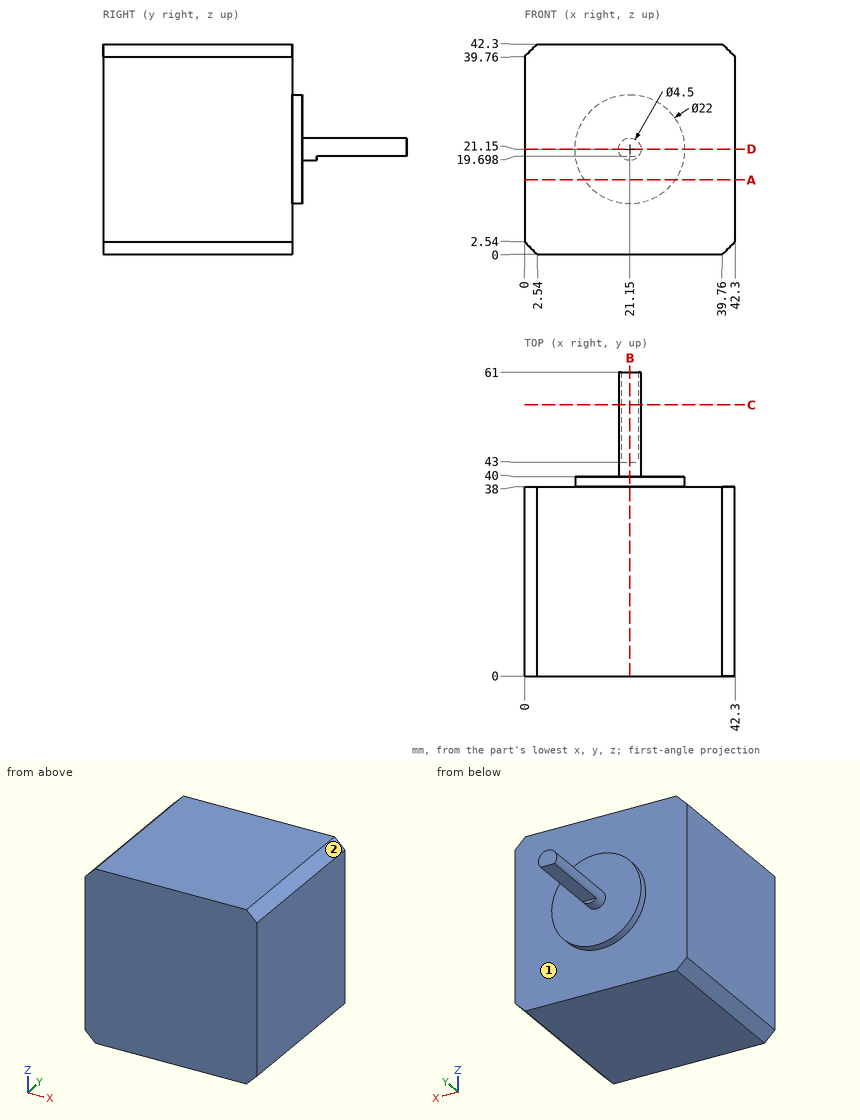
Study the drawing (mm; zero at the part's minimum x, y, z) and answer. A direction names the side the tool comes from. Give positions to 0.01 mm unless a question says otherwise; leave off trailing zeros. Write each loop counter-clockwise with the first axis right and the second up, starting at its lowest first coordinate (ties: lowest second). Pieces come first, ordered by that corner, then holes. Notation, with made-up numbers: (-3, -16.75) - (31, -16.75) arc R19 ccw to (31, 3.25) - close; hole circle Ø6 at (73, 63.5). An arc over 180 degrees is marked (long way). Use CSV: the item, a comma, the result in double quotes. Start each with the question number.
(1) Find section D-D (z = 21.15). Give the vertices of the cut face in (x, y).
(2) Consider line 1 along Y through (x, z) = (35, 4); line 2 along Y through (x, z) = (14, 14); line 3 along Z through (x, y) = (19.5, 54.5) (1 decimal). Determine where each line is inside the solid, lowest interval first.
(3) For the marked faces 1 and 2, determine the directions among +Z, -Z, +X, -X, +Y, -Y from which every point of the face is accessible in a straight line to the end or side of a thin tool.
(4) Find section A-A (z = 15). Give the vertices of the cut face in (x, y), plus the area to 3 significant figures.
(5) Given P1, Ø3, axis at x = 21.5, y = 51, coming from the +Z side; P2, Ø12, axis at x = 9, z = 6, coming from the +Y side; P3, Ø4, axis at x = 20.5, y = 53, coming from the -Z side, each flat-ended and moving along its own axis, determine where each tip first touches the part or whether it passes through.
(6) Find section C-C (y = 54.5). Give the vertices of the cut face in (x, z).
(7) Find section B-B (x = 21.15). Give the vertices of the cut face in (y, z).
Findings below:
1,outline,"(0, 0) - (42.3, 0) - (42.3, 38) - (32.15, 38) - (32.15, 40) - (23.4, 40) - (23.4, 61) - (18.9, 61) - (18.9, 40) - (10.15, 40) - (10.15, 38) - (0, 38) - close"
2,line 1,"0 to 38"
2,line 2,"0 to 40"
2,line 3,"19.7 to 22.7"
3,face 1,"+Y"
3,face 2,"+Z, +X, +Y, -Y"
4,outline,"(0, 0) - (42.3, 0) - (42.3, 38) - (30.27, 38) - (30.27, 40) - (12.03, 40) - (12.03, 38) - (0, 38) - close"
4,area,"1,640 mm2"
5,P1,"z = 23.4"
5,P2,"y = 38"
5,P3,"z = 19.7"
6,outline,"(19.43, 19.7) - (22.87, 19.7) arc R2.25 ccw (long way) to start"
7,outline,"(0, 0) - (38, 0) - (38, 10.15) - (40, 10.15) - (40, 18.9) - (43, 18.9) - (43, 19.7) - (61, 19.7) - (61, 23.4) - (40, 23.4) - (40, 32.15) - (38, 32.15) - (38, 42.3) - (0, 42.3) - close"
